Check sheet for the drawn part. Datum: minimum x, y, z corner. Units: mm. A direction names the side the tool comes from. Give positions to 0.01 mm unless a question says otherwise; leave off trailing zeros. Write each loop counter-clockwise with the first axis right and the second up, starting at its lowest first coordinate (ties: lowest second). Pieces come first, ordered by that corner, then holes.
(1) Cross-section at C-C (x = 85). Record the boundary of the cut face in (y, z), and give its area (3 significant figures).
(2) Cross-section at A-A (z = 27.5). Record the boundary of the cut face in (x, y), and give its area (3 significant figures).
(3) Tool access check on the marked faces 5, 6 and 7. Record the directions out of +Z, -Z, +X, -X, +Y, -Y that give a thin tool (end or side, any length) a straight path to the whole face; none if there is none.
(4) Cross-section at D-D (z = 74). Record the boundary of the cut face in (x, y), and give its area (3 significant figures).
(5) Depth check by flat-ended pin: P1, Ø4, axis at x = 16.5, y = 48, coming from the -Z side; P2, Ø1.5, axis at x = 54.5, z = 68.5, coming from the -Y side; P3, Ø22.5, axis at x = 52.5, y = 39, coming from the +Z side. Enter the tip coordinate at first touch or a pass-through.
(6) Mould release check, pull along X, two halves, no side actions. Record for the marked faces 1, 2, 3 and 4: +X half, -X half, draft (parallel to the pull), parting line (faces both ways), or undercut.
(7) Thickness scan on line 1 along X through (y, z) = (75.5, 39.5); line 2 along Z through (x, y) = (6, 67); line 3 along Y through (x, z) = (52, 90). Record the ranges inside material, lowest first.
(8) Cross-section at B-B (y = 30.5). Record the boundary of the cut face in (x, z), and give its area (3 significant figures).
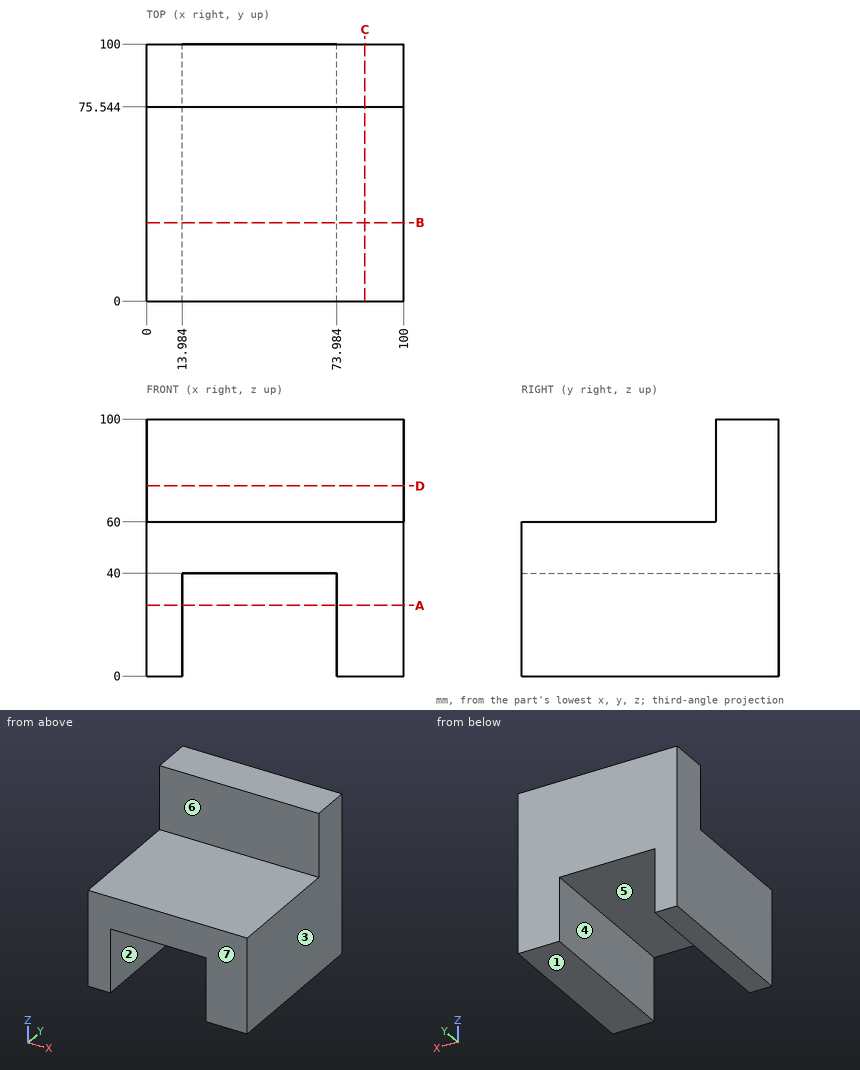
Reply:
1. outline: (0, 0) - (100, 0) - (100, 100) - (75.54, 100) - (75.54, 60) - (0, 60) - close
1. area: 6,980 mm2
2. outline: (0, 0) - (13.98, 0) - (13.98, 100) - (0, 100) - close; (73.98, 0) - (100, 0) - (100, 100) - (73.98, 100) - close
2. area: 4,000 mm2
3. face 5: -Z, +Y, -Y
3. face 6: +Z, +X, -X, -Y
3. face 7: +Z, -Z, +X, -X, -Y
4. outline: (0, 75.54) - (100, 75.54) - (100, 100) - (0, 100) - close
4. area: 2,450 mm2
5. P1: stops at z = 40
5. P2: stops at y = 75.54
5. P3: stops at z = 60
6. face 1: draft
6. face 2: undercut
6. face 3: +X half
6. face 4: undercut
7. line 1: x = 0 to 13.98, 73.98 to 100
7. line 2: z = 0 to 60
7. line 3: y = 75.54 to 100
8. outline: (0, 0) - (13.98, 0) - (13.98, 40) - (73.98, 40) - (73.98, 0) - (100, 0) - (100, 60) - (0, 60) - close
8. area: 3,600 mm2
